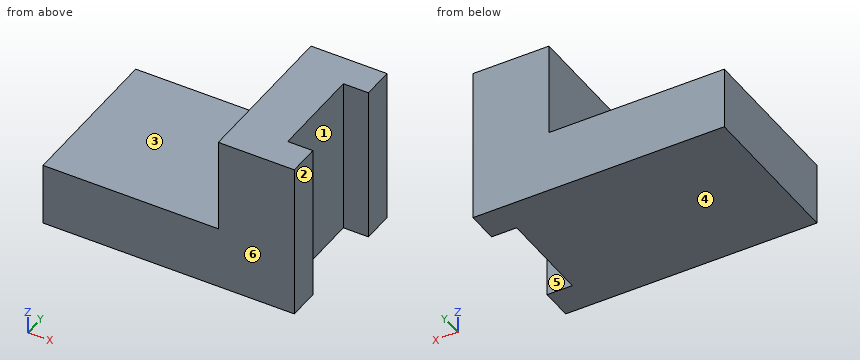
```python
from build123d import *

# Parameters (mm, degrees)
F0_W     = 55.8011086538
F0_H     = 50
F1_DEPTH = 20
F2_DEPTH = 50


with BuildPart() as f1:
    # F0 (on Top) → F1 (new body)
    with BuildSketch(Plane.XY):
        with Locations((27.9005543269, 25)):
            Rectangle(F0_W, F0_H)
    extrude(amount=F1_DEPTH)

    # F0 (on Top) → F2 (join)
    with BuildSketch(Plane.XY):
        Polygon((55.8011086538, 50), (55.8011086538, 0), (80, 0), (80, 10), (72, 10), (72, 40), (80, 40), (80, 50), align=None)
    extrude(amount=F2_DEPTH)


solid = f1.part
```
The listing builds one solid part. Answer for the finished solid, in the listing's coordinates (mm). Face numbers are marked on the shaded views. A direction names the side the tool comes from. Give positions to 0.01 mm unless a question says otherwise; leave off trailing zeros. Write each loop counter-clockwise with the first axis right and the second up, starting at its lowest first coordinate (ties: lowest second). Pieces come first, ordered by that corner, then holes. Notation, with made-up numbers: (17.5, 81) - (61.5, 81) arc R17 cw to (61.5, 105) - close; hole circle Ø8 at (87, -0.5). An arc over 180 degrees is marked (long way). Use one line per item in the form item = value. Start each with the question number.
1) Find section C-C on x = 13.5. Determine the outline of the cut face in (y, z), plus the area to 3 significant figures.
2) Find section A-A on y = 43.5. Determine the outline of the cut face in (x, z).
3) Flat-ended cylindrical pins translate along their axes: pin 1 Ø8 at (y, z) = (26.5, 18.5) entering from +X; pin 2 Ø25 at (x, y) = (40, 33) entering from +Z. Find the tip coordinate at first contact, or state that the pin passes through.
4) A tool of negligible diameter and unlimited length cuts with its end or side. For the marked faces 1, 2 and 3, from which of +Z, -Z, +X, -X, +Y, -Y can it reach the whole face along a straight path? Write none if from no direction.
5) Consider line 1 along Y through (x, z) = (76.5, 20.5); line 2 along X through (y, z) = (29, 31); line 3 along Z through (x, y) = (48.5, 32). Determine where each line is inside the solid, lowest interval first. Write a range as from..to.
6) The mould has two halves that part along Y. Classify the marked faces 4, 5 and 6: pulls with the +Y half, pulls with the -Y half, needs draft (parallel to the pull), parting line crosses it, or undercut.
7) Find section D-D on z = 26.5. Determine the outline of the cut face in (x, y), plus the area to 3 significant figures.
8) Find section B-B on z = 12.5. Determine the outline of the cut face in (x, y), plus the area to 3 significant figures.
Geometry results:
q1.outline = (0, 0) - (50, 0) - (50, 20) - (0, 20) - close
q1.area = 1,000 mm2
q2.outline = (0, 0) - (80, 0) - (80, 50) - (55.8, 50) - (55.8, 20) - (0, 20) - close
q3.pin_1 = 72
q3.pin_2 = 20
q4.face_1 = +Z, -Z, +X
q4.face_2 = +Z, -Z, +X, +Y, -Y
q4.face_3 = +Z, -X, +Y, -Y
q5.line_1 = 0..10, 40..50
q5.line_2 = 55.8..72
q5.line_3 = 0..20
q6.face_4 = needs draft
q6.face_5 = undercut
q6.face_6 = pulls with the -Y half
q7.outline = (55.8, 0) - (80, 0) - (80, 10) - (72, 10) - (72, 40) - (80, 40) - (80, 50) - (55.8, 50) - close
q7.area = 970 mm2
q8.outline = (0, 0) - (80, 0) - (80, 10) - (72, 10) - (72, 40) - (80, 40) - (80, 50) - (0, 50) - close
q8.area = 3,760 mm2
